```python
from build123d import *

# Parameters (mm, degrees)
SKETCH1_R                                     = 25
BOSS_EXTRUDE1_DEPTH                           = 5
CHAMFER1_SIZE                                 = 1
CSK_FOR_M4_COUNTERSUNK_FLAT_HEAD1_D           = 4.5
CSK_FOR_M4_COUNTERSUNK_FLAT_HEAD1_CSINK_D     = 9.4
CSK_FOR_M4_COUNTERSUNK_FLAT_HEAD1_CSINK_ANGLE = 90
M12X1_25_TAPPED_HOLE1_D                       = 10.8
M12X1_25_TAPPED_HOLE1_ON_FACE_2_D             = 10.8
CIRPATTERN1_COUNT                             = 3


with BuildPart() as part:
    # Sketch1 → Boss-Extrude1 (new body)
    with BuildSketch(Plane(origin=(0, 0, 0), x_dir=(1, 0, 0), z_dir=(0, 1, 0))):
        with Locations(Location((0, 0, 0), (0, 0, 270))):
            Circle(SKETCH1_R)
    extrude(amount=BOSS_EXTRUDE1_DEPTH)

    # Chamfer1
    chamfer1_edges = [part.edges().sort_by_distance(p)[0] for p in [
        (0, 5, -25),
    ]]
    chamfer(chamfer1_edges, length=CHAMFER1_SIZE)

    # CSK for M4 Countersunk Flat Head1 (through all)
    with Locations(Plane(origin=(0, 5, -18), x_dir=(0, 0, 1), z_dir=(0, 1, 0))):
        with Locations((0, 0)):
            csk_for_m4_countersunk_flat_head1 = CounterSinkHole(CSK_FOR_M4_COUNTERSUNK_FLAT_HEAD1_D / 2, CSK_FOR_M4_COUNTERSUNK_FLAT_HEAD1_CSINK_D / 2, counter_sink_angle=CSK_FOR_M4_COUNTERSUNK_FLAT_HEAD1_CSINK_ANGLE)

    # M12x1.25 Tapped Hole1 (through all)
    with Locations(Plane(origin=(0, 0, 0), x_dir=(0, 0, -1), z_dir=(0, -1, 0))):
        with Locations((0, 0)):
            Hole(M12X1_25_TAPPED_HOLE1_D / 2)

    # M12x1.25 Tapped Hole1 on face 2 (through all)
    with Locations(Plane.ZX.offset(5)):
        with Locations((0, 0)):
            Hole(M12X1_25_TAPPED_HOLE1_ON_FACE_2_D / 2)

    # CirPattern1: CSK for M4 Countersunk Flat Head1 ×3 about axis
    cirpattern1_axis = Axis((0, 0, 0), (0, 1, 0))
    for i in range(1, CIRPATTERN1_COUNT):
        add(csk_for_m4_countersunk_flat_head1.rotate(cirpattern1_axis, i * 360 / CIRPATTERN1_COUNT), mode=Mode.SUBTRACT)


solid = part.part
```
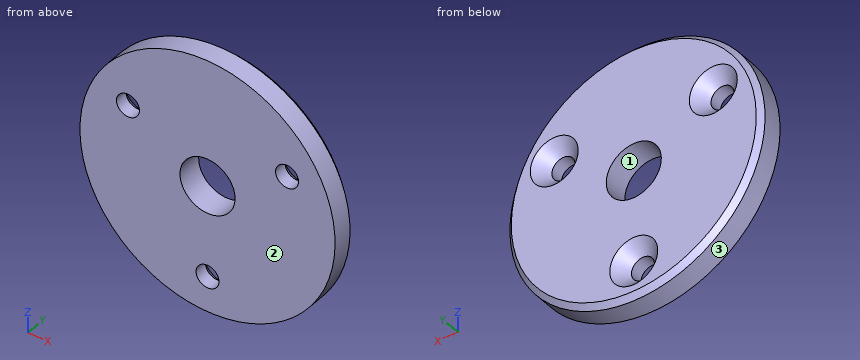
Model file for the job. Use its own axes, mm. Face numbers are marked on the shaded views. Coordinates: 2 decimals unless noted, no trailing zeros. Loops run counter-clockwise (first coordinate to the right, second up) from the corner with the lowest first, then second, coordinate; pieces in that order, holes last. Notation, with made-up numbers: M 85,-26.5 L 134,-26.5 A30 ccw 134,4.5 Z; hole C 21.5,-21 d6. An arc over 180 degrees is marked long. Use CSV: the item, a comma, the result in double quotes. Start each with the question number.
1. Band-saw the part on D-D, the plane z = 9. Give the number of separate pieces and of enclosed holes in the cut face, then the cut area to 3 significant figures.
2. Band-saw the part on C-C, the plane y = 0.7. List the corners of the cut face in (x, z) (3 decimals).
3. Two-plate mould, pull along Z, no slides. Class the marked faces 1, 2 and 3: pulls with the +Z half, pulls with the -Z half, needs draft (parallel to the pull), parting line crosses it, or undercut.
4. Band-saw the part on B-B, the plane x = 0. List the corners of the cut face in (y, z).
5. Probe probe 1 along X at (y, z) = (0.5, 9); probe 2 along X at (y, z) = (1.95, 7); probe 3 along Z at (x, y) = (2, 4.1). List the from-to ranges inside material, lowest first. Write a range as [from, to].
6. Flat gauge pins, fed straight in: pin 1 (5 mm diameter, centred on x = 0, z = -18, fed in from +Y); pin 2 (6 mm diameter, centred on x = -15.59, z = 9, fed in from +Y); pin 3 (3.5 mm diameter, centred on x = 15.59, z = 9, fed in from -Y); pin 4 (2 mm diameter, centred on y = 1.5, z = 10, fed in from +X). Where does each tip first touch, or does it go through?
7. Band-saw the part on A-A, the plane z = 0. List the corners of the cut face in (x, y), then the cut area to 3 significant figures.
Entries:
1,separate pieces,"3"
1,enclosed holes,"0"
1,area,"175 mm2"
2,outline,"C 0,0 d50; hole C -15.588,9 d4.5; hole C 0,0 d10.8; hole C 0,-18 d4.5; hole C 15.588,9 d4.5"
3,face 1,"undercut"
3,face 2,"needs draft"
3,face 3,"parting line crosses it"
4,outline,"M 0,-25 L 4,-25 L 5,-24 L 5,-22.7 L 2.55,-20.25 L 0,-20.25 Z; M 0,-15.75 L 2.55,-15.75 L 5,-13.3 L 5,-5.4 L 0,-5.4 Z; M 0,5.4 L 5,5.4 L 5,24 L 4,25 L 0,25 Z"
5,probe 1,"x = [-23.32, -17.84], [-13.34, 13.34], [17.84, 23.32]"
5,probe 2,"x = [-24, -16.62], [-14.56, 14.56], [16.62, 24]"
5,probe 3,"z = [-24.82, -21.23], [-14.77, -5.02], [5.02, 24.82]"
6,pin 1,"stops at y = 2.8"
6,pin 2,"stops at y = 3.3"
6,pin 3,"passes through"
6,pin 4,"stops at x = 23.32"
7,outline,"M -25,0 L -5.4,0 L -5.4,5 L -24,5 L -25,4 Z; M 5.4,0 L 25,0 L 25,4 L 24,5 L 5.4,5 Z"
7,area,"195 mm2"
